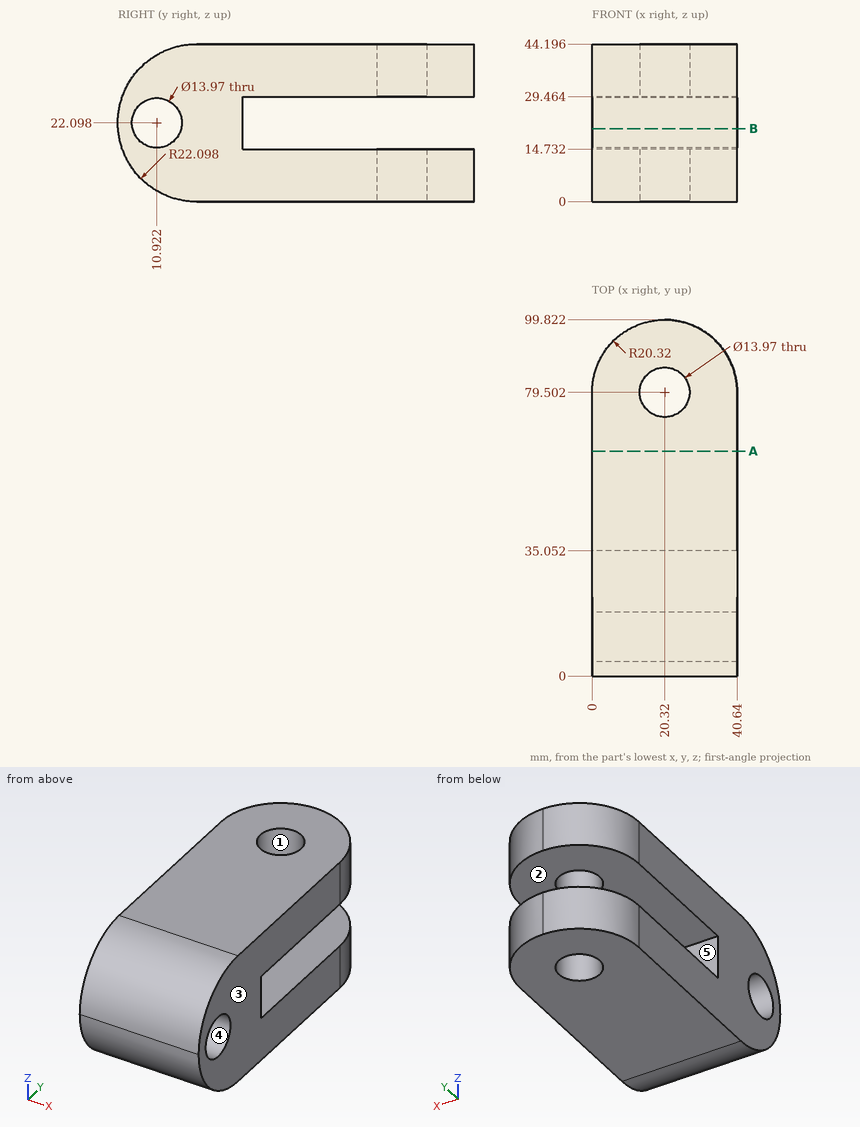
Here's the drawing with two shaded views (mm, measured from the low corner). I have some questions. A direction names the side the tool comes from. Give positions to 0.01 mm unless a question says otherwise; leave off trailing zeros. Write each loop counter-clockwise with the first axis right and the second up, starting at its lowest first coordinate (ties: lowest second). Pieces come first, ordered by that corner, then holes. Notation, with made-up numbers: (84.5, -22) -> (111.5, -22) arc R27 cw to (111.5, -3) -> close; hole circle Ø5 at (-13.5, -8.75). An arc over 180 degrees is marked (long way). Use one line per item in the form item = value. Start each with the question number.
1. Imagine slicing it at A-A on y = 63. List the corners of the cut face in (x, z) for me.
2. Thinking about a two-plate mould opening in X: for the marked faces 1, 2 and 3, which applies, +X half, -X half, draft (parallel to the pull), parting line (faces both ways), or undercut?
3. On a 3-axis mill with a long thin cutter (end or side, diameter ignored), from which of +Z, -Z, +X, -X, +Y, -Y can I reach the whole of each face in a straight line? I mean the marked faces 4 and 5. Say none if no direction works.
4. Imagine slicing it at B-B on z = 20.5. List the corners of the cut face in (x, y) for me, plus the area to 3 significant figures.
5. If I drill on L1, parallel to Z at x = 4, y = 45; L2, parallel to Y at x = 6, z = 17; L3, parallel to Y at x = 36, z = 28.5, over which ranges is the centre line in solid material (lowest first)?
6. Will this pin go through, and if not, where does the flat tip stop? pin 1 Ø4 at (x, z) = (6.5, 25.5) entering from +Y.
Entries:
q1.outline = (0, 0) -> (40.64, 0) -> (40.64, 14.73) -> (0, 14.73) -> close; (0, 29.46) -> (40.64, 29.46) -> (40.64, 44.2) -> (0, 44.2) -> close
q2.face_1 = undercut
q2.face_2 = draft
q2.face_3 = +X half
q3.face_4 = +X, -X
q3.face_5 = +X, -X, +Y
q4.outline = (0, 0.06) -> (40.64, 0.06) -> (40.64, 4.12) -> (0, 4.12) -> close; (0, 17.72) -> (40.64, 17.72) -> (40.64, 35.05) -> (0, 35.05) -> close
q4.area = 869 mm²
q5.L1 = 0 to 14.73, 29.46 to 44.2
q5.L2 = 0.6 to 6.15, 15.7 to 35.05
q5.L3 = 0.95 to 8.13, 13.72 to 35.05
q6.pin_1 = 35.05
